Here's how the part is built. I have some questions about the finished solid (model axes, mm). Round coordinates to 2 decimals unless told otherwise and drop trailing zeros. Order: outer loops, then holes, each group sorted by start corner. A loop starts at its lowest first (then second) coordinate and runs counter-clockwise, first axis right, second up. Notation, with made-up numbers: M 75,-34 L 128,-34 A29 cw 128,-3 Z; hole C -26,87.5 d8. An arc over 180 degrees is marked long. Write item = value, one per line. Start each with the question number.
Item 1: I want a section at C-C, the plane x = -8.15. List the corners of the cut face in (y, z) for me.
Item 2: I want a section at B-B, the plane x = -6.85. List the corners of the cut face in (y, z) for me, plus the area to 3 significant figures.
Item 3: I want a section at D-D, the plane x = -4.55. List the corners of the cut face in (y, z) for me, plus the area to 3 significant figures.
Item 4: I'm going to push flat-ended pins straight in: P1, Ø5, axis at y = -63.5, z = 10, coming from the -X side; P2, Ø1, axis at x = -5, y = -59.5, coming from the +Z side; P3, Ø1.5, axis at x = -8, y = -62.5, coming from the +Z side. Where does each tip first touch, or does it pass through?
Item 5: Please list where these lines run through material, in increasing order: L1, parallel to Y at x = -5.95, z = 7; L2, parallel to Y at x = -7.05, z = 10; L3, parallel to Y at x = -7.15, z = 8.75.
Item 6: I want a section at A-A, the plane x = -6.2. List the corners of the cut face in (y, z) for me.
Item 7: We'd pull the mould along X, two halves only. Please class faces 1 (the face through (-6.52, -68.64, 12.81)), 2 (the face through (-6.51, -59.971, 5.885)), 3 (the face through (-5.231, -58.811, 6.407)): pulls with the +X half, pulls with the -X half, needs draft (parallel to the pull), parting line crosses it, or undercut.
```python
from build123d import *

# Parameters (mm, degrees)
SKETCH020_R             = 2.75
PAD008_DEPTH            = 3
SKETCH001_R             = 1.5
PAD009_DEPTH            = 10
POCKET011_DEPTH         = 4
BODY003_PLACEMENT_ANGLE = 225


with BuildPart() as part:
    # Sketch020 → Pad008 (new body)
    with BuildSketch(Plane.XY):
        Circle(SKETCH020_R)
    extrude(amount=PAD008_DEPTH)

    # Sketch001 (on Face2 of Pad008) → Pad009 (join)
    with BuildSketch(Plane(origin=(0, 0, 0), x_dir=(1, 0, 0), z_dir=(0, 0, -1))):
        Circle(SKETCH001_R)
    extrude(amount=PAD009_DEPTH)

    # Sketch021 (on DatumPlane) → Pocket011 (cut)
    with BuildSketch(Plane.XY.offset(3)):
        Polygon((0.721688, -1.25), (1.443376, 0), (0.721688, 1.25), (-0.721688, 1.25), (-1.443376, 0), (-0.721688, -1.25), align=None)
    extrude(amount=-POCKET011_DEPTH, mode=Mode.SUBTRACT)


with BuildPart() as part_1:
    # Body003 placement: moved
    add(part.part.moved(Location((-6.5, -61.581981, 5.727565))).rotate(Axis((-6.5, -61.581981, 5.727565), (1, 0, 0)), BODY003_PLACEMENT_ANGLE))


solid = part_1.part
```
Filled in:
q1.outline = M -63.14,4.17 L -61.02,2.05 L -57.91,5.16 L -60.03,7.28 Z
q2.outline = M -69.68,11.77 L -62.61,4.7 L -63.51,3.8 L -61.39,1.68 L -60.34,2.72 L -63.17,5.55 L -61.41,7.32 L -58.58,4.49 L -57.53,5.53 L -59.65,7.66 L -60.55,6.76 L -67.62,13.83 Z
q2.area = 35.5 mm^2
q3.outline = M -62.95,4.36 L -60.83,2.24 L -58.09,4.98 L -60.21,7.1 Z
q3.area = 11.6 mm^2
q4.P1 = -8
q4.P2 = 7.51
q4.P3 = 8.8
q5.L1 = -64.83 to -61.72, -61.09 to -60.88, -60.31 to -59.04
q5.L2 = -67.83 to -63.88
q5.L3 = -66.52 to -62.69
q6.outline = M -69.69,11.76 L -62.62,4.69 L -63.51,3.79 L -61.39,1.67 L -60.34,2.72 L -63.17,5.55 L -61.41,7.32 L -58.58,4.49 L -57.53,5.54 L -59.65,7.66 L -60.54,6.77 L -67.61,13.84 Z
q7.face_1 = needs draft
q7.face_2 = undercut
q7.face_3 = parting line crosses it
